Read the model definition and answer for the solid it produces. Units are mm, in the model's axes. A direction names the side the tool comes from. Give positions to 0.01 mm unless a question says otherwise; leave off trailing zeros. Write each loop counter-clockwise with the first axis right and the second up, starting at its lowest first coordinate (ties: lowest second). Pieces come first, ordered by that corner, then holes.
```python
from build123d import *

# Parameters (mm, degrees)
SKETCH5_R           = 5
BOSS_EXTRUDE2_DEPTH = 5
SKETCH6_R           = 17.5
BOSS_EXTRUDE3_DEPTH = 1.5
SKETCH7_R           = 1.7
CUT_EXTRUDE1_DEPTH  = 7
FILLET1_R           = 10


with BuildPart() as part:
    # Sketch3 → Revolve1 (revolve)
    with BuildSketch(Plane.XY, mode=Mode.PRIVATE) as revolve1_sk:
        Polygon((0, 0), (2.5, 0), (5, 5), (0, 5), align=None)
    revolve(revolve1_sk.sketch.rotate(Axis((0, 0, 0), (0, 1, 0)), 90), axis=Axis((0, 0, 0), (0, 1, 0)))

    # Sketch5 → Boss-Extrude2 (add)
    with BuildSketch(Plane(origin=(0, 5, 0), x_dir=(1, 0, 0), z_dir=(0, 1, 0))):
        with Locations(Location((0, 0, 0), (0, 0, 270))):
            Circle(SKETCH5_R)
    extrude(amount=BOSS_EXTRUDE2_DEPTH)

    # Sketch6 → Boss-Extrude3 (add)
    with BuildSketch(Plane(origin=(0, 10, 0), x_dir=(1, 0, 0), z_dir=(0, 1, 0))):
        with Locations(Location((0, 0, 0), (0, 0, 270))):
            Circle(SKETCH6_R)
    extrude(amount=BOSS_EXTRUDE3_DEPTH)

    # Sketch7 → Cut-Extrude1 (cut)
    with BuildSketch(Plane.XZ):
        with Locations(Location((0, 0, 0), (0, 0, 270))):
            Circle(SKETCH7_R)
    extrude(amount=-CUT_EXTRUDE1_DEPTH, mode=Mode.SUBTRACT)

    # Fillet1
    # the kernel refuses this fillet: 10 mm, written as the material it adds along each edge
    with BuildSketch(Plane(origin=(0, 10, 0), x_dir=(0, 0, 1), z_dir=(-1, 0, 0))) as fillet1_piece_1:
        with BuildLine():
            CenterArc((13.660254038, -10), FILLET1_R, 90, 60)
            Line((5, -5), (4.826794919, -4.9))
            ThreePointArc((4.826794919, -4.9), (4.8, -2.5), (4.8, 0))
            Line((4.8, 0), (5, 0.2))
            Line((5, 0.2), (13.660254038, 0.2))
            Line((13.660254038, 0.2), (13.660254038, 0))
        make_face()
    revolve(axis=Axis((0, 10, 0), (0, 1, 0)))


solid = part.part
```
Item 1: Section C-C (y = 10.5) is taken. Write down the section's boundary in (x, z).
Result set:
outline: circle Ø35 at (0, 0)
Item 2: Section D-D (y = 4.25) is taken. Write down the section's boundary in (x, z) (3 decimals), and give its area (3 significant figures).
Result set:
outline: circle Ø9.25 at (0, 0); hole circle Ø3.4 at (0, 0)
area: 58.1 mm2
Item 3: Determine the mould class of faces 1 (the flat face through (0, 7, 0)), 2 (the flat face through (1, 0, 2)), 3 (the cylindrical face through (-1.66, 3.45, 0.37)), 4 (the conical face through (2.864, 0.868, 0.636)) for opening direction Z: pulls with the +Z half, pulls with the -Z half, needs draft (parallel to the pull), parting line crosses it, or undercut.
Result set:
face 1: undercut
face 2: needs draft
face 3: undercut
face 4: parting line crosses it
Item 4: Which of the six approach directions +Z, -Z, +X, -X, +Y, -Y give full straight-line access (tool end or side, diameter ignored) to faces 5 (the flat face through (0, 11.5, 0)), 6 (the flat face through (-10.3, 10, -9.2))?
Result set:
face 5: +Z, -Z, +X, -X, +Y
face 6: -Y
Item 5: Find the intervals of material crossed by line 1 along X through (y, z) = (4.5, 0); line 2 along X through (y, z) = (1.5, 0); line 3 along Y through (x, z) = (5, -15), in increasing order.
Result set:
line 1: x = -4.75 to -1.7, 1.7 to 4.75
line 2: x = -3.25 to -1.7, 1.7 to 3.25
line 3: y = 10 to 11.5
Item 6: Section B-B (x = 0) is taken. Write down the section's boundary in (y, z).
Result set:
outline: (0, -2.5) - (5, -5) arc R10 cw to (10, -13.66) - (10, -17.5) - (11.5, -17.5) - (11.5, 17.5) - (10, 17.5) - (10, 13.66) arc R10 cw to (5, 5) - (0, 2.5) - (0, 1.7) - (7, 1.7) - (7, -1.7) - (0, -1.7) - close
Item 7: Section A-A (z = 0) is taken. Write down the section's boundary in (x, y).
Result set:
outline: (-17.5, 10) - (-13.66, 10) arc R10 cw to (-5, 5) - (-2.5, 0) - (-1.7, 0) - (-1.7, 7) - (1.7, 7) - (1.7, 0) - (2.5, 0) - (5, 5) arc R10 cw to (13.66, 10) - (17.5, 10) - (17.5, 11.5) - (-17.5, 11.5) - close
Item 8: Each of these flat-tipped pins is pushed along its axis until it touches: pin 1 Ø5 at (x, y) = (7, 10) entering from -Z; pin 2 Ø1.7 at (x, z) = (-0.5, -0.5) entering from -Y; pin 3 Ø12 at (x, z) = (-12.5, 3.5) entering from -Y. Where does it stop, or does it pass through?
Result set:
pin 1: stops at z = -16.91
pin 2: stops at y = 7
pin 3: stops at y = 7.44
